Job drawing, mm, ordinate dimensions from the low corner. One solid piece. A direction names the side the tool comes from. Round coordinates to 2 decimals unless told otherwise and drop trailing zeros. Loops run counter-clockwise (first coordinate to the right, second up) from the corner with the lowest first, then second, coordinate; pieces in that order, holes last. Notation, with made-up numbers: M 25,31.25 L 82,31.25 A33 ccw 82,64.25 Z; hole C 59.5,55.5 d1. An arc over 180 degrees is marked long. Use one line per item in the form item = value.
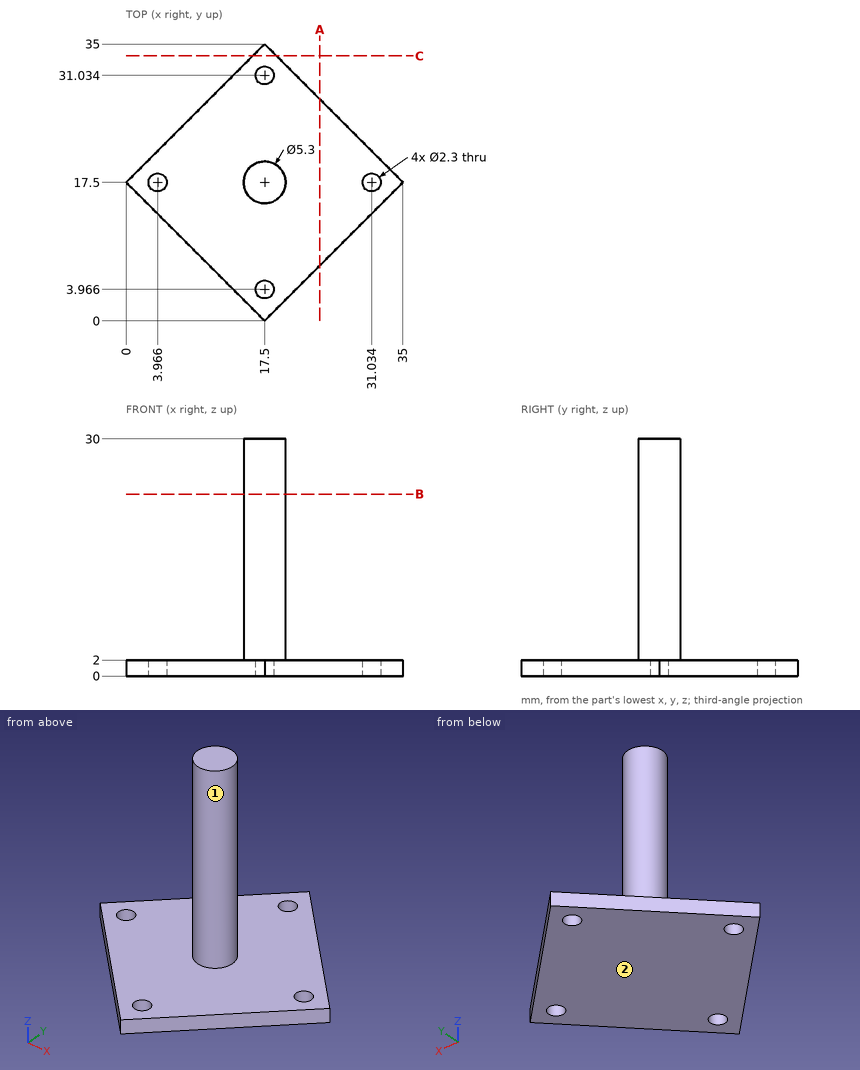
1. Tool access for the marked faces 1 and 2: list every direction of +Z, -Z, +X, -X, +Y, -Y with a clear straight run to the whole face (end or side of a thin tool).
Completed:
face_1 = +Z
face_2 = -Z, +X, -X, +Y, -Y
2. Probe line 1 along Z through (x, y) = (19, 8); line 2 along X through (y, z) = (17, 3.5). List the from-to ranges inside material, lowest first. Write a range as from..to.
Completed:
line_1 = 0..2
line_2 = 14.9..20.1
3. Cut at B-B on z = 23. Write the cut outline in (x, y).
Completed:
outline = C 17.5,17.5 d5.3
4. Cut at A-A on x = 24.5. Write the cut outline in (y, z), and give its area (3 significant figures).
Completed:
outline = M 7,0 L 28,0 L 28,2 L 7,2 Z
area = 42.0 mm2
5. Drop flat-ended pins along their axis: P1, Ø8, axis at y = 17, z = 13.5, coming from the +X side; P2, Ø2.5, axis at x = 31.03, y = 17.5, coming from the -Z side; P3, Ø3, axis at x = 26.5, y = 29.5, coming from the +Z side; P4, Ø6, axis at y = 18, z = 14, coming from the -X side. Give the stop position or say it passes through.
Completed:
P1 = 20.15
P2 = 0
P3 = through
P4 = 14.85
6. Cut at C-C on y = 33.5. Write the cut outline in (x, z).
Completed:
outline = M 16,0 L 19,0 L 19,2 L 16,2 Z
